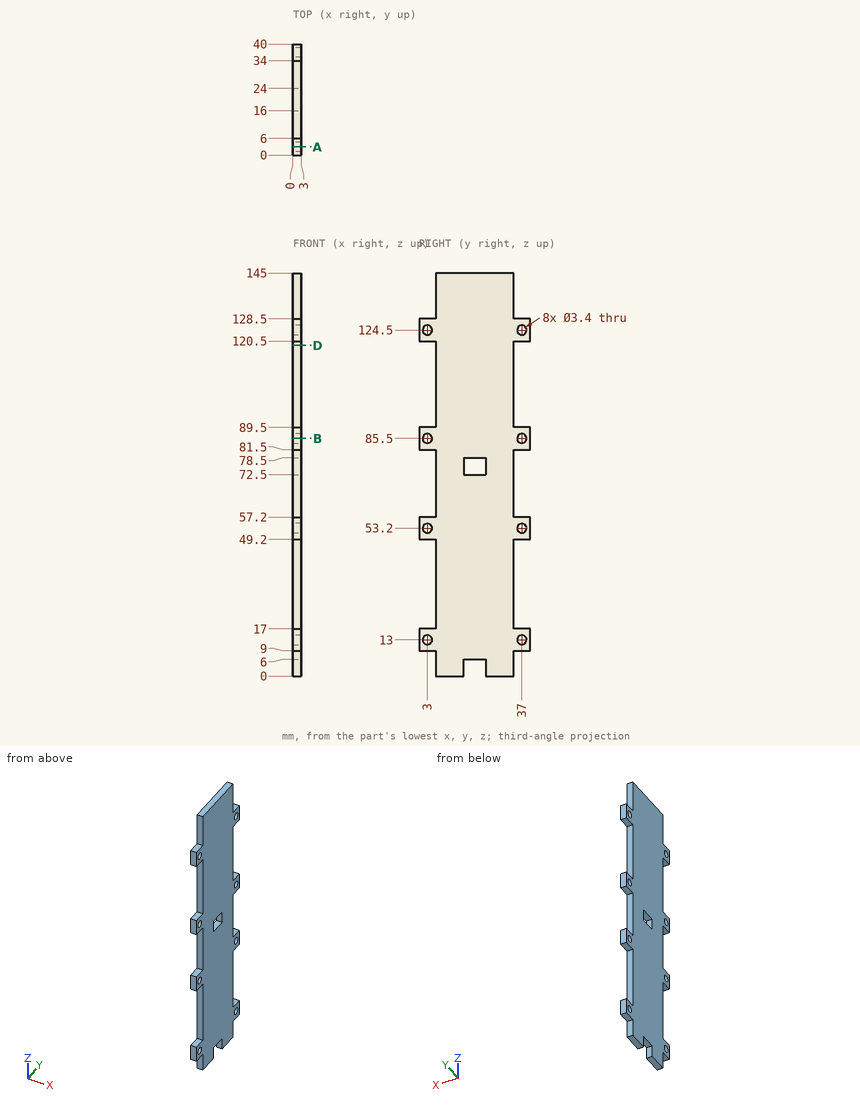
Design review of the part shown in the three views and the two pictorial views. Dimensions are in mm from the part's minimum x, y and z. Give positions to 0.01 mm unless a question says otherwise; leave off trailing zeros. Loops run counter-clockwise (first coordinate to the right, second up) from the corner with the lowest first, then second, coordinate; pieces in that order, holes last. Notation, with made-up numbers: (56.25, 44.5) -> (101.25, 44.5) arc R32 cw to (101.25, 82.5) -> close; hole circle Ø6 at (-30.5, 11). An arc over 180 degrees is marked (long way). Write each question's results on one line, items separated by ' | '.
Q1. Take a section at D-D, the plane z = 119. Write out the cut boundary in (x, y).
Reply:
outline: (0, 6) -> (3, 6) -> (3, 34) -> (0, 34) -> close
Q2. Wall thickness on L1, parallel to Y at x = 1.1, z = 53.2; L2, parallel to Z at x = 2.65, y = 20.5; L3, parallel to Y at x = 2.4, z = 24: over which ranges is each line inside the solid? List them lowest first.
Reply:
L1: y = 0 to 1.3, 4.7 to 35.3, 38.7 to 40 | L2: z = 6 to 72.5, 78.5 to 145 | L3: y = 6 to 34
Q3. Take a section at B-B, the plane z = 85.5. Write out the cut boundary in (x, y), plus the area to 3 significant figures.
Reply:
outline: (0, 0) -> (3, 0) -> (3, 1.3) -> (0, 1.3) -> close; (0, 4.7) -> (3, 4.7) -> (3, 35.3) -> (0, 35.3) -> close; (0, 38.7) -> (3, 38.7) -> (3, 40) -> (0, 40) -> close | area: 99.6 mm²
Q4. For pin 1 Ø0.9 at (x, y) = (1.5, 2.5) entering from -Z; pin 2 Ø4.5 at (y, z) = (37, 124.5) entering from -X; pin 3 Ø1.5 at (x, z) = (1.5, 110.5) entering from -Y; pin 4 Ø2.5 at (y, z) = (37, 85.5) entering from -X, all flat-tipped, find the tip position at first contact; note any pin that passes through.
Reply:
pin 1: stops at z = 9 | pin 2: stops at x = 0 | pin 3: stops at y = 6 | pin 4: passes through
Q5. Take a section at A-A, the plane y = 3. Give the number of separate pieces and of enclosed holes in the cut face, plus the area to 3 significant figures.
Reply:
separate pieces: 8 | enclosed holes: 0 | area: 55.2 mm²
